For this review, take the finished solid that the model builds, in its own axes (mm). A direction names the side the tool comes from. Round coordinates to 2 decimals unless told otherwise and drop trailing zeros. Order: outer loops, then holes, each group sorted by start corner. A loop starts at its lowest first (then second) coordinate and runs counter-clockwise, first axis right, second up. Notation, with made-up numbers: (-33.5, 85.5) -> (5.5, 85.5) arc R20 ccw to (5.5, 107.5) -> close; hole circle Ø3 at (85, 10). An arc over 180 degrees is marked (long way). Use a Markdown table: item, result. Add a question column.
1) Machinability: for faces 1 (the face through (32.959, 1.565, 26.224)), 2 (the face through (29, 3.175, 31)), which of the approach directions +Z, -Z, +X, -X, +Y, -Y give a long, thin tool a straight path to every point of the face, cutting with its end or side? Answer none if there is none.
2) Consider section B-B (z = 37.5). State the section outline as (x, y) points (3 decimals).
3) Clearance check with flat-ended pins moving along their axes: P1, Ø10, axis at x = 27.5, z = 34.5, coming from the +Y side (3 decimals); P2, Ø13.5, axis at x = 22.81, z = 25.4, coming from the +Y side; P3, Ø24, axis at y = 20, z = 25.5, coming from the -X side (3 decimals). State where each tip first meets the part, or that it passes through.
4) Consider section D-D (z = 8). State the section outline as (x, y) points (3 decimals), plus the area to 4 significant figures.
5) Draft analysis for pull direction X (two halves, no side actions). For faces 3 (the face through (16.46, 1.57, 34.86)), 4 (the face through (50.8, 14, 19)), 5 (the face through (37, 3, 50.8)), state which applies: pulls with the +X half, pulls with the -X half, needs draft (parallel to the pull), parting line crosses it, or undercut.
6) Consider section C-C (x = 20.5). State the section outline as (y, z) points (3 decimals).
7) Wall thickness on line 1 along Y through (x, z) = (49, 25); line 2 along X through (y, z) = (48, 39) (3 decimals); line 3 along Y through (x, z) = (30, 14) (3 decimals): over which ranges is each line inside the solid? List them lowest first. Write a range as [from, to].
8) Consider section A-A (y = 31). State the section outline as (x, z) points (1 decimal).
```python
from build123d import *

# Parameters (mm, degrees)
BOSS_EXTRUDE1_DEPTH = 50.8
SKETCH2_R           = 14.2875
CUT_EXTRUDE1_DEPTH  = 50.8
SKETCH3_R           = 7.62
CUT_EXTRUDE2_DEPTH  = 50.8
SKETCH4_R           = 1.7859375
CUT_EXTRUDE3_DEPTH  = 12.7


with BuildPart() as part:
    # Sketch1 → Boss-Extrude1 (new body)
    with BuildSketch(Plane.XY):
        Polygon((0, 3.175), (0, 0), (47.625, 0), (50.8, 0), (50.8, 3.175), (50.8, 50.8), (47.625, 50.8), (47.625, 3.175), align=None)
    extrude(amount=BOSS_EXTRUDE1_DEPTH)

    # Sketch2 → Cut-Extrude1 (cut)
    with BuildSketch(Plane.ZY.offset(-47.625)):
        with Locations((25.4, 26.9875)):
            Circle(SKETCH2_R)
    extrude(amount=-CUT_EXTRUDE1_DEPTH, mode=Mode.SUBTRACT)

    # Sketch3 → Cut-Extrude2 (cut)
    with BuildSketch(Plane(origin=(0, 3.175, 0), x_dir=(1, 0, 0), z_dir=(0, 1, 0))):
        with Locations(Location((22.8092, -25.4, 0), (0, 0, 270))):
            Circle(SKETCH3_R)
    extrude(amount=-CUT_EXTRUDE2_DEPTH, mode=Mode.SUBTRACT)

    # Sketch4 → Cut-Extrude3 (cut)
    with BuildSketch(Plane.XZ):
        with Locations(Location((15.250391474, 33.54567799, 0), (0, 0, 270))):
            Circle(SKETCH4_R)
        with Locations(Location((19.534240193, 14.781040799, 0), (0, 0, 270))):
            Circle(SKETCH4_R)
        with Locations(Location((33.642968333, 27.873281211, 0), (0, 0, 270))):
            Circle(SKETCH4_R)
    extrude(amount=-CUT_EXTRUDE3_DEPTH, mode=Mode.SUBTRACT)


solid = part.part
```
Results list:
| question | item | result |
|---|---|---|
| 1 | face 1 | +Y, -Y |
| 1 | face 2 | +Z, -Z, -X, +Y |
| 2 | outline | (0, 0) -> (50.8, 0) -> (50.8, 19.39) -> (47.625, 19.39) -> (47.625, 3.175) -> (0, 3.175) -> close; (47.625, 34.585) -> (50.8, 34.585) -> (50.8, 50.8) -> (47.625, 50.8) -> close |
| 3 | P1 | y = 3.175 |
| 3 | P2 | through |
| 3 | P3 | x = 47.625 |
| 4 | outline | (0, 0) -> (50.8, 0) -> (50.8, 50.8) -> (47.625, 50.8) -> (47.625, 3.175) -> (0, 3.175) -> close |
| 4 | area | 312.5 mm2 |
| 5 | face 3 | undercut |
| 5 | face 4 | pulls with the +X half |
| 5 | face 5 | needs draft |
| 6 | outline | (0, 0) -> (3.175, 0) -> (3.175, 13.279) -> (0, 13.279) -> close; (0, 16.283) -> (3.175, 16.283) -> (3.175, 18.138) -> (0, 18.138) -> close; (0, 32.662) -> (3.175, 32.662) -> (3.175, 50.8) -> (0, 50.8) -> close |
| 7 | line 1 | [0, 12.71], [41.27, 50.8] |
| 7 | line 2 | [47.625, 50.8] |
| 7 | line 3 | [0, 3.175] |
| 8 | outline | (47.6, 0) -> (50.8, 0) -> (50.8, 11.7) -> (47.6, 11.7) -> close; (47.6, 39.1) -> (50.8, 39.1) -> (50.8, 50.8) -> (47.6, 50.8) -> close |
